Read the model definition and answer for the solid it produces. Units are mm, in the model's axes. Give positions to 0.01 mm unless a question says otherwise; leave off trailing zeros. Loops run counter-clockwise (first coordinate to the right, second up) from the corner with the lowest first, then second, coordinate; pieces in that order, holes last.
(1) Find section A-A, the plane x = -100. Write down the section's boundary in (y, z), then the cut area to 3 significant figures.
(2) Find section B-B, the plane z = 73. Write down the section's boundary in (x, y).
(3) Find section C-C, the plane y = 14.75. Write down the section's boundary in (x, z), then the cut area to 3 significant figures.
(4) Each of these flat-tipped pins is pushed along its axis until it touches: P1, Ø9, axis at x = -216.5, y = 12.5, coming from the +Z side; P2, Ø5.5, axis at x = -220, y = 13, coming from the -Z side; P3, Ø2.5, axis at y = 9, z = 109.7, coming from the +X side. Where does it stop, or does it pass through?
(5) Find section D-D, the plane z = 47. Write down the section's boundary in (x, y), then the cut area to 3 significant figures.
(6) Straight lines are drawn through the part: probe 1 along X at (y, z) = (2.75, 86); probe 2 along X at (y, z) = (4.25, 82); probe 3 along Z at (x, y) = (100, 9.75). For each, find the intervals that lie inside material, in ascending order.
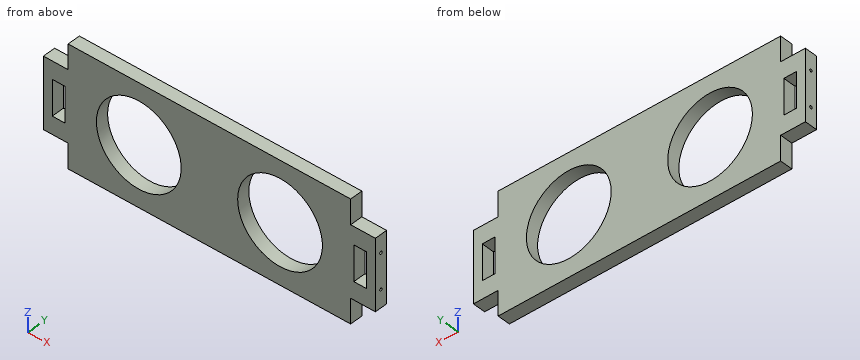
Autodesk Inventor part; units mm, degrees
ref_plane "YZ Plane" through (0, 0, 0) normal (1, 0, 0) x (0, 1, 0)
ref_plane "XZ Plane" through (0, 0, 0) normal (0, 1, 0) x (-1, 0, 0)
ref_plane "XY Plane" through (0, 0, 0) normal (0, 0, 1) x (1, 0, 0)
sketch "Boceto1" plane through (0, 0, 0) normal (0, 1, 0) x (-1, 0, 0)
  line L0 (200, 169.7039) -> (-200, 169.7039)
  line L1 (-235, 134.7039) -> (-235, 34.7039)
  line L2 (-200, -0.2961) -> (200, -0.2961)
  line L3 (235, 34.7039) -> (235, 134.7039)
  circle A0 centre (100, 85) radius 60
  line L4 (222.5, 109.7039) -> (204.5, 109.7039)
  line L5 (204.5, 109.7039) -> (204.5, 59.7039)
  line L6 (204.5, 59.7039) -> (222.5, 59.7039)
  line L7 (222.5, 59.7039) -> (222.5, 109.7039)
  line L8 (235, 134.7039) -> (200, 134.7039)
  line L9 (200, 134.7039) -> (200, 169.7039)
  line L10 (235, 34.7039) -> (200, 34.7039)
  line L11 (200, 34.7039) -> (200, -0.2961)
  line L12 (-235, 34.7039) -> (-235, 134.7039)
  circle A1 centre (-100, 85) radius 60
  line L13 (-222.5, 109.7039) -> (-204.5, 109.7039)
  line L14 (-204.5, 109.7039) -> (-204.5, 59.7039)
  line L15 (-204.5, 59.7039) -> (-222.5, 59.7039)
  line L16 (-222.5, 59.7039) -> (-222.5, 109.7039)
  line L17 (-235, 134.7039) -> (-200, 134.7039)
  line L18 (-200, 134.7039) -> (-200, 169.7039)
  line L19 (-235, 34.7039) -> (-200, 34.7039)
  line L20 (-200, 34.7039) -> (-200, -0.2961)
  point P0 (0, 0)
  point P1 (235, 84.7039)
  point P2 (217.5, 134.7039)
  point P3 (-235, 84.7039)
  point P4 (-217.5, 134.7039)
  dimension "d4" = 120
  dimension "d5" = 18
  dimension "d6" = 35
  dimension "d7" = 35
  dimension "d8" = 35
  dimension "d9" = 50
  dimension "d10" = 25
  dimension "d11" = 12.5
  dimension "d12" = 100
  dimension "d15" = 470
  dimension "d16" = 12.5
  dimension "d17" = 18
extrude "Extrusión1" add sketch "Boceto1" along normal blind 18
sketch "Boceto2" plane through (235, 0, 134.7039) normal (1, 0, 0) x (0, 0, -1)
  circle A0 centre (75, 9) radius 2
  circle A1 centre (25, 9) radius 2
  line L0 (0, 0) -> (100, 0)
  line L1 (0, 0) -> (0, 18)
  point P0 (134.7039, 0)
  dimension "d18" = 4
  dimension "d19" = 4
  dimension "d20" = 9
  dimension "d21" = 9
  dimension "d22" = 25
  dimension "d23" = 50
extrude "Extrusión2" cut sketch "Boceto2" against normal blind 10
sketch "Boceto3" plane through (-235, 0, 34.7039) normal (-1, 0, 0) x (0, 0, 1)
  circle A0 centre (25, 9) radius 2
  circle A1 centre (25, 9) radius 2
  circle A2 centre (75, 9) radius 2
  circle A3 centre (75, 9) radius 2
  point P0 (-34.7039, 0)
  dimension "d26" = 4
  dimension "d27" = 4
extrude "Extrusión3" cut sketch "Boceto3" against normal blind 10
properties part number "APM_001-2"
Entries:
1. outline: (0, -0.3) - (18, -0.3) - (18, 25) - (0, 25) - close; (0, 145) - (18, 145) - (18, 169.7) - (0, 169.7) - close
1. area: 900 mm2
2. outline: (-235, 0) - (-222.5, 0) - (-222.5, 18) - (-235, 18) - close; (-204.5, 0) - (-158.79, 0) - (-158.79, 18) - (-204.5, 18) - close; (-41.21, 0) - (41.21, 0) - (41.21, 18) - (-41.21, 18) - close; (158.79, 0) - (204.5, 0) - (204.5, 18) - (158.79, 18) - close; (222.5, 0) - (235, 0) - (235, 18) - (222.5, 18) - close
3. outline: (-235, 34.7) - (-200, 34.7) - (-200, -0.3) - (200, -0.3) - (200, 34.7) - (235, 34.7) - (235, 134.7) - (200, 134.7) - (200, 169.7) - (-200, 169.7) - (-200, 134.7) - (-235, 134.7) - close; hole (-222.5, 59.7) - (-204.5, 59.7) - (-204.5, 109.7) - (-222.5, 109.7) - close; hole circle Ø120 at (-100, 85); hole circle Ø120 at (100, 85); hole (204.5, 59.7) - (222.5, 59.7) - (222.5, 109.7) - (204.5, 109.7) - close
3. area: 50,600 mm2
4. P1: stops at z = 134.7
4. P2: stops at z = 34.7
4. P3: stops at x = 225
5. outline: (-235, 0) - (-146.43, 0) - (-146.43, 18) - (-235, 18) - close; (-53.57, 0) - (53.57, 0) - (53.57, 18) - (-53.57, 18) - close; (146.43, 0) - (235, 0) - (235, 18) - (146.43, 18) - close
5. area: 5,120 mm2
6. probe 1: x = -235 to -222.5, -204.5 to -159.99, -40.01 to 40.01, 159.99 to 204.5, 222.5 to 235
6. probe 2: x = -235 to -222.5, -204.5 to -159.92, -40.08 to 40.08, 159.92 to 204.5, 222.5 to 235
6. probe 3: z = -0.3 to 25, 145 to 169.7
